```python
from build123d import *

# Parameters (mm, degrees)
BOSS_EXTRUDE1_DEPTH = 50.8
CUT_EXTRUDE1_DEPTH  = 3.175
SKETCH3_R           = 3.429
CUT_EXTRUDE2_DEPTH  = 66.068137364
SKETCH5_R           = 3.429
CUT_EXTRUDE4_DEPTH  = 108.200338152
CUT_EXTRUDE9_START  = 38.1
CUT_EXTRUDE9_DEPTH  = 3.175
SKETCH11_OUTSIDE_W  = 89.994
SKETCH11_OUTSIDE_H  = 51.894
TRIM_DEPTH          = 108.200338152


with BuildPart() as part:
    # Sketch1 → Boss-Extrude1 (new, symmetric)
    with BuildSketch(Plane.XY):
        Polygon((-25.4, 6.35), (-25.4, 12.7), (25.4, 12.7), (25.4, 6.35), (31.75, 0), (25.4, -6.35), (25.4, -12.7), (-25.4, -12.7), (-25.4, -6.35), (-31.75, 0), align=None)
    extrude(amount=BOSS_EXTRUDE1_DEPTH, both=True)

    # Sketch2 → Cut-Extrude1 (cut, symmetric)
    with BuildSketch(Plane(origin=(0, 0, 0), x_dir=(1, 0, 0), z_dir=(0, 1, 0))):
        Polygon((48.874015971, 6.39418036), (12.7, 6.39418036), (7.239, 9.54709018), (7.239, 15.85290982), (12.7, 19.00581964), (48.874015971, 19.00581964), align=None)
        Polygon((48.874015971, -19.00581964), (12.7, -19.00581964), (7.239, -15.85290982), (7.239, -9.54709018), (12.7, -6.39418036), (48.874015971, -6.39418036), align=None)
        Polygon((7.239, 34.94709018), (12.7, 31.79418036), (48.874015971, 31.79418036), (48.874015971, 44.40581964), (12.7, 44.40581964), (7.239, 41.25290982), align=None)
        Polygon((48.874015971, -44.40581964), (12.7, -44.40581964), (7.239, -41.25290982), (7.239, -34.94709018), (12.7, -31.79418036), (48.874015971, -31.79418036), align=None)
        Polygon((-7.239, -34.94709018), (-7.239, -41.25290982), (-12.7, -44.40581964), (-48.874015971, -44.40581964), (-48.874015971, -31.79418036), (-12.7, -31.79418036), align=None)
        Polygon((-48.874015971, -6.39418036), (-48.874015971, -19.00581964), (-12.7, -19.00581964), (-7.239, -15.85290982), (-7.239, -9.54709018), (-12.7, -6.39418036), align=None)
        Polygon((-48.874015971, 31.79418036), (-12.7, 31.79418036), (-7.239, 34.94709018), (-7.239, 41.25290982), (-12.7, 44.40581964), (-48.874015971, 44.40581964), align=None)
        Polygon((-48.874015971, 19.00581964), (-48.874015971, 6.39418036), (-12.7, 6.39418036), (-7.239, 9.54709018), (-7.239, 15.85290982), (-12.7, 19.00581964), align=None)
    extrude(amount=CUT_EXTRUDE1_DEPTH, both=True, mode=Mode.SUBTRACT)

    # Sketch3 → Cut-Extrude2 (cut, through all)
    with BuildSketch(Plane(origin=(0, 12.7, 0), x_dir=(1, 0, 0), z_dir=(0, 1, 0))):
        with Locations(Location((-12.7, 38.1, 0), (0, 0, 180))):
            Circle(SKETCH3_R)
        with Locations(Location((12.7, 38.1, 0), (0, 0, 180))):
            Circle(SKETCH3_R)
        with Locations(Location((12.7, 12.7, 0), (0, 0, 180))):
            Circle(SKETCH3_R)
        with Locations(Location((-12.7, 12.7, 0), (0, 0, 180))):
            Circle(SKETCH3_R)
        with Locations(Location((-12.7, -12.7, 0), (0, 0, 180))):
            Circle(SKETCH3_R)
        with Locations(Location((12.7, -12.7, 0), (0, 0, 180))):
            Circle(SKETCH3_R)
        with Locations(Location((-12.7, -38.1, 0), (0, 0, 180))):
            Circle(SKETCH3_R)
        with Locations(Location((12.7, -38.1, 0), (0, 0, 180))):
            Circle(SKETCH3_R)
    extrude(amount=-CUT_EXTRUDE2_DEPTH, mode=Mode.SUBTRACT)

    # Sketch5 → Cut-Extrude4 (cut, through all)
    with BuildSketch(Plane.XY.offset(50.8)):
        Circle(SKETCH5_R)
    extrude(amount=-CUT_EXTRUDE4_DEPTH, mode=Mode.SUBTRACT)

    # Sketch10 → Cut-Extrude9 (cut, symmetric)
    with BuildSketch(Plane.XY.offset(CUT_EXTRUDE9_START)):
        Polygon((3.15290982, -5.461), (6.30581964, 0), (6.30581964, 55.166180444), (-6.30581964, 55.166180444), (-6.30581964, 0), (-3.15290982, -5.461), align=None)
    cut_extrude9 = extrude(amount=CUT_EXTRUDE9_DEPTH, both=True, mode=Mode.SUBTRACT)

    # Mirror1: Cut-Extrude9 across plane
    add(cut_extrude9.mirror(Plane.XY), mode=Mode.SUBTRACT)

    # Sketch11 outside → Trim (cut, through all)
    with BuildSketch(Plane.XY.offset(50.8)):
        Rectangle(SKETCH11_OUTSIDE_W, SKETCH11_OUTSIDE_H)
        Polygon((-24.892, 12.7), (-24.892, 6.13957951), (-31.03157951, 0), (-24.892, -6.13957951), (-24.892, -12.7), (24.892, -12.7), (24.892, -6.13957951), (31.03157951, 0), (24.892, 6.13957951), (24.892, 12.7), align=None, mode=Mode.SUBTRACT)
    extrude(amount=-TRIM_DEPTH, mode=Mode.SUBTRACT)


solid = part.part
```
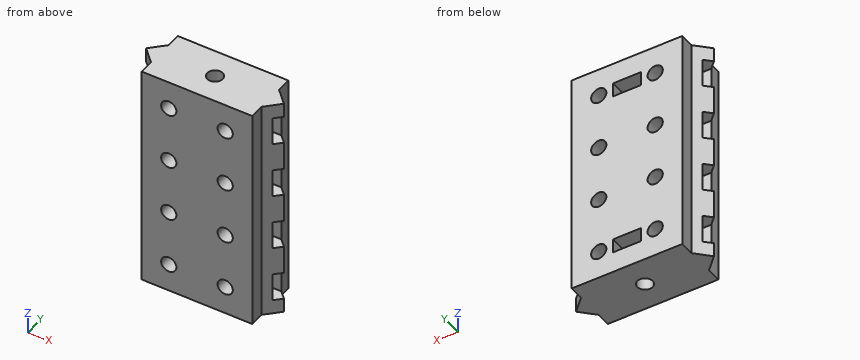
Model file for the job. Use its own axes, mm. Round coordinates to 2 decimals unless told otherwise and drop trailing zeros. Write each loop counter-clockwise with the first axis right and the second up, starting at its lowest first coordinate (ties: lowest second). Pieces come first, ordered by that corner, then holes. Notation, with made-up numbers: (29.5, -23.75) - (71.5, -23.75) arc R22 cw to (71.5, 5.25) - close; hole circle Ø5 at (72, 73.25). An arc over 180 degrees is marked (long way). One line per item, written item: value.
(1) Cut at C-C, the plane x = 19.5. Give the cut face in (y, z) (3 decimals), plus the area to 3 significant figures.
Values follow:
outline: (-12.7, -50.8) - (12.7, -50.8) - (12.7, 50.8) - (-12.7, 50.8) - close; hole (-3.175, -44.406) - (3.175, -44.406) - (3.175, -31.794) - (-3.175, -31.794) - close; hole (-3.175, -19.006) - (3.175, -19.006) - (3.175, -6.394) - (-3.175, -6.394) - close; hole (-3.175, 6.394) - (3.175, 6.394) - (3.175, 19.006) - (-3.175, 19.006) - close; hole (-3.175, 31.794) - (3.175, 31.794) - (3.175, 44.406) - (-3.175, 44.406) - close
area: 2,260 mm²
(2) Cut at D-D, the plane z = -38.1. Give the number of separate pieces and of enclosed holes in the cut face, plus the area to 3 significant figures.
Values follow:
separate pieces: 5
enclosed holes: 0
area: 585 mm²
(3) Wall check: probe 1 along X at (y, z) = (-10.75, -13); probe 2 along Z at (x, y) = (-0.5, -4.25) (3 decimals); probe 3 along Z at (x, y) = (12.7, 9.75). Give the ranges that are in metal, low to high.
Values follow:
probe 1: x = -24.89 to -16.12, -9.28 to 9.28, 16.12 to 24.89
probe 2: z = -50.8 to -41.275, -34.925 to 34.925, 41.275 to 50.8
probe 3: z = -50.8 to -41.53, -34.67 to -16.13, -9.27 to 9.27, 16.13 to 34.67, 41.53 to 50.8
(4) Cut at B-B, the plane x = 0. Give the cut face in (y, z) (3 decimals).
Values follow:
outline: (-12.7, -50.8) - (-3.429, -50.8) - (-3.429, -41.275) - (-5.461, -41.275) - (-5.461, -34.925) - (-3.429, -34.925) - (-3.429, 34.925) - (-5.461, 34.925) - (-5.461, 41.275) - (-3.429, 41.275) - (-3.429, 50.8) - (-12.7, 50.8) - close; (3.429, -50.8) - (12.7, -50.8) - (12.7, -41.275) - (3.429, -41.275) - close; (3.429, -34.925) - (12.7, -34.925) - (12.7, 34.925) - (3.429, 34.925) - close; (3.429, 41.275) - (12.7, 41.275) - (12.7, 50.8) - (3.429, 50.8) - close
(5) Drop flat-ended pins along their axis: P1, Ø5, axis at y = -9.5, z = 7.5, coming from the +X side; P2, Ø1.5, axis at y = 9.5, z = -28.5, coming from the -X side; P3, Ø7, axis at y = 5, z = 37, coming from the +X side. Give the stop position or say it passes through.
Values follow:
P1: stops at x = 24.89
P2: stops at x = -24.89
P3: stops at x = 27.86
(6) Cut at A-A, the plane z = 0.5. Give the cut face in (x, y), plus the area to 3 significant figures.
Values follow:
outline: (-31.03, 0) - (-24.89, -6.14) - (-24.89, -12.7) - (24.89, -12.7) - (24.89, -6.14) - (31.03, 0) - (24.89, 6.14) - (24.89, 12.7) - (-24.89, 12.7) - (-24.89, 6.14) - close; hole circle Ø6.86 at (0, 0)
area: 1,300 mm²
